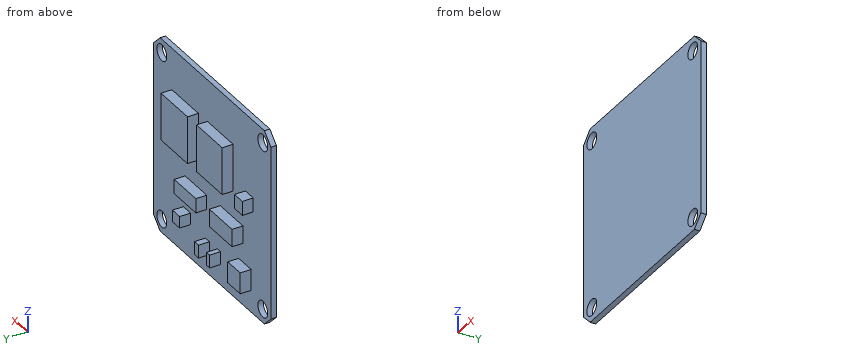
```python
from build123d import *

# Parameters (mm, degrees)
SKETCH1_W            = 36
SKETCH1_H            = 36
BOSS_EXTRUDE1_DEPTH  = 1
SKETCH2_W            = 3.81533948
SKETCH2_H            = 3.898281644
SKETCH2_W_2          = 7.879505449
SKETCH2_H_2          = 8.708927076
SKETCH2_W_3          = 8.128331937
SKETCH2_W_4          = 6.63537301
SKETCH2_H_3          = 2.654149204
SKETCH2_W_5          = 6.967141661
SKETCH2_H_4          = 3.234744343
SKETCH2_W_6          = 0.958696997
SKETCH2_H_5          = 2.396742492
SKETCH2_W_7          = 1.244132439
BOSS_EXTRUDE2_DEPTH  = 2
CHAMFER1_SIZE        = 2
SKETCH3_W            = 2.408590064
SKETCH3_H            = 2.601230853
SKETCH3_W_2          = 2.217469356
SKETCH3_H_2          = 2.137281434
BOSS_EXTRUDE3_DEPTH  = 2
SKETCH4_R            = 1.5
CUT_EXTRUDE1_DEPTH   = 2
LPATTERN1_COUNT      = 2
LPATTERN1_PITCH      = 31
LPATTERN1_COUNT_DIR2 = 2
LPATTERN1_PITCH_DIR2 = 31


with BuildPart() as part:
    # Sketch1 → Boss-Extrude1 (new body)
    with BuildSketch(Plane(origin=(0, 0, 0), x_dir=(1, 0, 0), z_dir=(0, 1, 0))):
        Rectangle(SKETCH1_W, SKETCH1_H)
    extrude(amount=BOSS_EXTRUDE1_DEPTH)

    # Sketch2 → Boss-Extrude2 (add)
    with BuildSketch(Plane(origin=(0, 1, 0), x_dir=(1, 0, 0), z_dir=(0, 1, 0))):
        with Locations((-10, 12)):
            Rectangle(SKETCH2_W, SKETCH2_H)
        with Locations((-2.446793798, -5.909629087)):
            Rectangle(SKETCH2_W_2, SKETCH2_H_2)
        with Locations((8.335687344, -5.909629087)):
            Rectangle(SKETCH2_W_3, SKETCH2_H_2)
        with Locations((5.018000839, 4.914323135)):
            Rectangle(SKETCH2_W_4, SKETCH2_H_3)
        with Locations((-5.930364628, 4.914323136)):
            Rectangle(SKETCH2_W_5, SKETCH2_H_4)
        with Locations((-2.06525985, 13.001183991)):
            Rectangle(SKETCH2_W_6, SKETCH2_H_5)
        with Locations((1.492958928, 13.001183991)):
            Rectangle(SKETCH2_W_7, SKETCH2_H_5)
    extrude(amount=BOSS_EXTRUDE2_DEPTH)

    # Chamfer1
    chamfer1_edges = [part.edges().sort_by_distance(p)[0] for p in [
        (18, 0.5, 18),
        (-18, 0.5, 18),
        (-18, 0.5, -18),
        (18, 0.5, -18),
    ]]
    chamfer(chamfer1_edges, length=CHAMFER1_SIZE)

    # Sketch3 → Boss-Extrude3 (add)
    with BuildSketch(Plane(origin=(0, 1, 0), x_dir=(1, 0, 0), z_dir=(0, 1, 0))):
        with Locations((-11.367372892, -2.320698042)):
            Rectangle(SKETCH3_W, SKETCH3_H)
        with Locations((7.776721419, 10.675684916)):
            Rectangle(SKETCH3_W_2, SKETCH3_H_2)
    extrude(amount=BOSS_EXTRUDE3_DEPTH)

    # Sketch4 → Cut-Extrude1 (cut, through all)
    with BuildSketch(Plane(origin=(0, 1, 0), x_dir=(1, 0, 0), z_dir=(0, 1, 0))):
        with Locations((-15.5, 15.5)):
            Circle(SKETCH4_R)
    cut_extrude1 = extrude(amount=-CUT_EXTRUDE1_DEPTH, mode=Mode.SUBTRACT)

    # LPattern1: Cut-Extrude1 2 × 2
    with Locations(*[(i * LPATTERN1_PITCH, 0, j * LPATTERN1_PITCH_DIR2) for i in range(LPATTERN1_COUNT) for j in range(LPATTERN1_COUNT_DIR2) if (i, j) != (0, 0)]):
        add(cut_extrude1, mode=Mode.SUBTRACT)


solid = part.part
```
Geometry check sheet. Reference: the model listing, model coordinates, mm. Coordinates: 2 decimals unless noted, no trailing zeros. Write each loop counter-clockwise with the first axis right and the second up, starting at its lowest first coordinate (ties: lowest second). Pieces come first, ordered by that corner, then holes. Notation, with made-up numbers: M 82,42.25 L 89,42.25 A15 cw 89,70.25 Z; hole C 26,25 d11. An arc over 180 degrees is marked long. One line per item, written item: value. Start each with the question number.
(1) Sectioned sample at B-B, the plane z = 15.5. Enter the section's corners in (x, y).
(2) Sectioned sample at D-D, the plane y = 1.65. State how many separate pieces and enclosed holes the cut face has, and give its area (3 significant figures).
(3) Sectioned sample at C-C, the plane x = 9.5. Enter the section's corners in (y, z).
(4) Sectioned sample at A-A, the plane x = 15.5. Enter the section's corners in (y, z), and give its area (3 significant figures).
(5) Scan lines: line 1 along X through (y, z) = (0.7, -15.5); line 2 along Z through (x, y) = (-3, 1.6). Record each from-to range of solid material in increasing order. Write a range as [from, to].
(6) Depth check by flat-ended pin: pin 1 (1.6 mm diameter, centred on y = 2, z = 6.5, fed in from +X); pin 2 (1 mm diameter, centred on x = 8.5, z = 1, fed in from +Y); pin 3 (0.6 mm diameter, centred on x = -3.5, y = 1.5, fed in from +Z). Enter the tip coordinate at first touch or a pass-through.
Filled sheet:
1. outline: M -18,0 L -17,0 L -17,1 L -18,1 Z; M -14,0 L 14,0 L 14,1 L -14,1 Z; M 17,0 L 18,0 L 18,1 L 17,1 Z
2. separate pieces: 9
2. enclosed holes: 0
2. area: 211 mm²
3. outline: M 0,-18 L 1,-18 L 1,1.56 L 3,1.56 L 3,10.26 L 1,10.26 L 1,18 L 0,18 Z
4. outline: M 0,-18 L 1,-18 L 1,-17 L 0,-17 Z; M 0,-14 L 1,-14 L 1,14 L 0,14 Z; M 0,17 L 1,17 L 1,18 L 0,18 Z
4. area: 30.0 mm²
5. line 1: [-18, -17], [-14, 14], [17, 18]
5. line 2: [-6.53, -3.3], [1.56, 10.26]
6. pin 1: x = 12.4
6. pin 2: y = 1
6. pin 3: z = 10.26
